from build123d import *

# Parameters (mm, degrees)
SKETCH1_R           = 15.24
BOSS_EXTRUDE1_DEPTH = 152.4
SKETCH2_R           = 16.51
BOSS_EXTRUDE2_DEPTH = 2.54


with BuildPart() as part:
    # Sketch1 → Boss-Extrude1 (new, symmetric)
    with BuildSketch(Plane.XY):
        with Locations(Location((0, 0, 0), (0, 0, 180))):
            Circle(SKETCH1_R)
    extrude(amount=BOSS_EXTRUDE1_DEPTH, both=True)

    # Sketch2 → Boss-Extrude2 (add)
    with BuildSketch(Plane.XY.offset(152.4)):
        Circle(SKETCH2_R)
    boss_extrude2 = extrude(amount=-BOSS_EXTRUDE2_DEPTH)

    # Mirror1: Boss-Extrude2 across plane
    add(boss_extrude2.mirror(Plane.XY))


solid = part.part
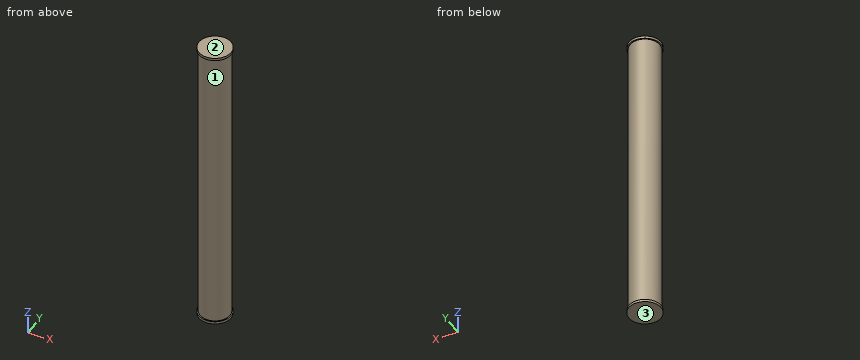
Verification items for the finished model (mm, model axes). Face numbers are marked on the shaded views. Coordinates: 2 decimals unless noted, no trailing zeros. Order: outer loops, then holes, each group sorted by start corner. A loop starts at its lowest first (then second) coordinate and runs counter-clockwise, first axis right, second up.
Item 1: Material ranges on L1, parallel to Z at x = 13, y = -10; L2, parallel to Y at x = 1, z = 128, recorded low to high.
Filled in:
L1: z = -152.4 to -149.86, 149.86 to 152.4
L2: y = -15.21 to 15.21
Item 2: Section check C-C, the plane z = 41. Enter the section's corners in (x, y), then the cut area to 3 significant figures.
Filled in:
outline: circle Ø30.48 at (0, 0)
area: 730 mm2
Item 3: Release check for a two-part mould opening along Z. For the marked faces 1, 2 and 3 record: +Z half, -Z half, draft (parallel to the pull), parting line (faces both ways), or undercut.
Filled in:
face 1: undercut
face 2: +Z half
face 3: -Z half
Item 4: Section check A-A, the plane x = 0. Enter the section's corners in (y, z), then the cut area to 3 significant figures.
Filled in:
outline: (-16.51, -152.4) - (16.51, -152.4) - (16.51, -149.86) - (15.24, -149.86) - (15.24, 149.86) - (16.51, 149.86) - (16.51, 152.4) - (-16.51, 152.4) - (-16.51, 149.86) - (-15.24, 149.86) - (-15.24, -149.86) - (-16.51, -149.86) - close
area: 9,300 mm2
Item 5: Depth check by flat-ended pin: pin 1 (10 mm diameter, centred on y = 4.5, z = 50.5, fed in from -X); pin 2 (5 mm diameter, centred on y = -4.5, z = -97.5, fed in from -X); pin 3 (8 mm diameter, centred on y = 13, z = -3.5, fed in from +X). Enter the tip coordinate at first touch or a pass-through.
Filled in:
pin 1: stops at x = -15.24
pin 2: stops at x = -15.11
pin 3: stops at x = 12.3
